```python
from build123d import *

# Parameters (mm, degrees)
F0_W     = 40
F0_H     = 80
F1_DEPTH = 20
F2_R     = 10
F3_DEPTH = 10
F5_W     = 20
F5_H     = 40
F6_DEPTH = 40
F7_R     = 10
F8_DEPTH = 40
F9_R     = 20
F10_R    = 19.99999


# Not quite as in the source:
# - a fillet or chamfer is up to 0.001 mm smaller than in the source, because OpenCascade refuses the exact size


with BuildPart() as f1:
    # F0 (on Right) → F1 (new body)
    with BuildSketch(Plane.YZ):
        with Locations((20, 40)):
            Rectangle(F0_W, F0_H)
    extrude(amount=F1_DEPTH)

    # F2 (on face) → F3 (join)
    with BuildSketch(Plane.YZ.offset(20)):
        with BuildLine():
            Line((0, 100), (0, 80))
            Line((0, 80), (40, 80))
            Line((40, 80), (40, 100))
            ThreePointArc((40, 100), (20, 120), (0, 100))
        make_face()
        with Locations((20, 100)):
            Circle(F2_R, mode=Mode.SUBTRACT)
    extrude(amount=-F3_DEPTH)

    # F4: F1 across face


with BuildPart() as f1_1:
    add(f1.part)
    add(f1.part.mirror(Plane(origin=(0, 20, 40), x_dir=(0, 1, 0), z_dir=(-1, 0, 0))))

    # F5 (on face) → F6 (cut, through all)
    with BuildSketch(Plane(origin=(0, 40, 0), x_dir=(-1, 0, 0), z_dir=(0, 1, 0))):
        with Locations((0, 20)):
            Rectangle(F5_W, F5_H)
    extrude(amount=-F6_DEPTH, mode=Mode.SUBTRACT)

    # F7 (on face) → F8 (cut, through all)
    with BuildSketch(Plane.YZ.offset(20)):
        with Locations((20, 20)):
            Circle(F7_R)
    extrude(amount=-F8_DEPTH, mode=Mode.SUBTRACT)

    # F9
    f9_edges = [f1_1.edges().sort_by_distance(p)[0] for p in [
        (-15, 0, 0),
    ]]
    fillet(f9_edges, radius=F9_R)

    # F10 (radius 20 in the source; OpenCascade refuses exactly that, so slightly less here)
    f10_edges = [f1_1.edges().sort_by_distance(p)[0] for p in [
        (-15, 40, 0),
        (15, 40, 0),
        (15, 0, 0),
    ]]
    fillet(f10_edges, radius=F10_R)


solid = f1_1.part
```
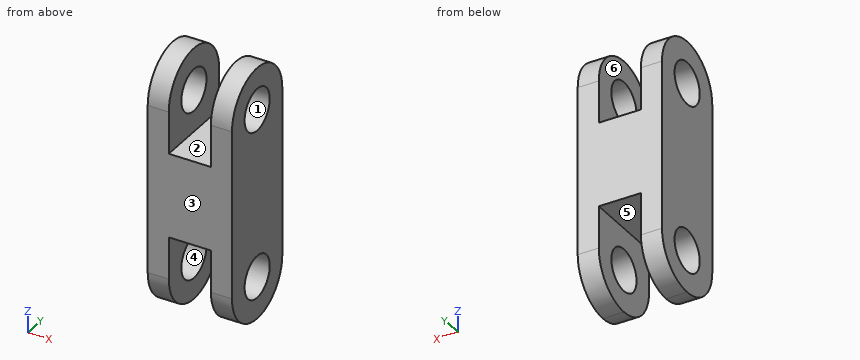
Model file for the job. Use its own axes, mm. Face numbers are marked on the shaded views. A direction names the side the tool comes from. Coordinates: 2 decimals unless noted, no trailing zeros. Order: outer loops, then holes, each group sorted by start corner. A loop starts at its lowest first (then second) coordinate and runs counter-clockwise, first axis right, second up. Notation, with made-up numbers: M 51,-9.75 L 76,-9.75 A20 cw 76,-4.75 Z; hole C -29,-4.5 d11. An arc over 180 degrees is marked long. Answer as CSV lines item,"result".
(1) Flat gauge pins, fed straight in: pin 1 (12 mm diameter, centred on y = 20, z = 100, fed in from -X); pin 2 (10 mm diameter, centred on x = 10, y = 7.5, fed in from -Z); pin 3 (3 mm diameter, centred on x = 3, y = 17, fed in from -Z); pin 4 (16 mm diameter, centred on x = 2.5, y = 25, fed in from +Z). Where does each tip first touch, or does it go through?
Geometry says:
pin 1,"passes through"
pin 2,"stops at z = 1.46"
pin 3,"stops at z = 40"
pin 4,"stops at z = 119.88"
(2) Band-saw the part on A-A, the plane y = 13. List the corners of the cut face in (x, z) (3 decimals), then the cut area to 3 significant figures.
Geometry says:
outline,"M -20,1.265 L -10,1.265 L -10,12.859 L -20,12.859 Z; M -20,27.141 L -10,27.141 L -10,40 L 10,40 L 10,27.141 L 20,27.141 L 20,92.859 L 10,92.859 L 10,80 L -10,80 L -10,92.859 L -20,92.859 Z; M -20,107.141 L -10,107.141 L -10,118.735 L -20,118.735 Z; M 10,1.265 L 20,1.265 L 20,12.859 L 10,12.859 Z; M 10,107.141 L 20,107.141 L 20,118.735 L 10,118.735 Z"
area,"2,580 mm2"
(3) Band-saw the part on D-D, the plane x = -1. List the corners of the cut face in (y, z).
Geometry says:
outline,"M 0,40 L 40,40 L 40,80 L 0,80 Z"
(4) Wall check: line 1 along Z through (x, y) = (13.5, 20); line 2 along X through (y, z) = (31.5, 20); line 3 along Z through (x, y) = (-5.5, 12.5). Give the ranges that are in metal, low to high.
Geometry says:
line 1,"z = 0 to 10, 30 to 90, 110 to 120"
line 2,"x = -20 to -10, 10 to 20"
line 3,"z = 40 to 80"
(5) Band-saw the part on C-C, the plane z = 26. List the corners of the cut face in (x, y).
Geometry says:
outline,"M -20,0 L -10,0 L -10,12 L -20,12 Z; M -20,28 L -10,28 L -10,40 L -20,40 Z; M 10,0 L 20,0 L 20,12 L 10,12 Z; M 10,28 L 20,28 L 20,40 L 10,40 Z"
(6) Band-saw the part on B-B, the plane x = 11.5. State how many separate pieces and enclosed holes the cut face has, then the cut area to 3 significant figures.
Geometry says:
separate pieces,"1"
enclosed holes,"2"
area,"3,830 mm2"
(7) Pull direction Z, two halves, no side cores. Call the marked faces 1, 2 and 3: +Z half, -Z half, draft (parallel to the pull), parting line (faces both ways), or undercut.
Geometry says:
face 1,"undercut"
face 2,"+Z half"
face 3,"draft"
(8) 3-axis set-ups, long thin cutter, end or side, ignore diameter. For the marked faces 4, 5 and 6: which of +Z, -Z, +X, -X, +Y, -Y reach the whole face in a straight line?
Geometry says:
face 4,"+X, -X"
face 5,"-Z, +Y, -Y"
face 6,"+Z, +Y, -Y"
